```python
from build123d import *

# Parameters (mm, degrees)
F1_DEPTH = 12.7
F2_SIZE  = 2.54


with BuildPart() as f1:
    # F0 (on Top) → F1 (new body)
    with BuildSketch(Plane.XY):
        Polygon((0, 76.2), (0, 0), (50.8, 0), (50.8, 55.88), (25.4, 76.2), align=None)
        Polygon((-50.8, 0), (0, 0), (0, 76.2), (-25.4, 76.2), (-50.8, 55.88), align=None)
        Polygon((0, -76.2), (0, 0), (-50.8, 0), (-50.8, -55.88), (-25.4, -76.2), align=None)
        Polygon((50.8, 0), (0, 0), (0, -76.2), (25.4, -76.2), (50.8, -55.88), align=None)
    extrude(amount=F1_DEPTH)

    # F2
    f2_edges = [f1.edges().sort_by_distance(p)[0] for p in [
        (50.8, 0, 0),
        (38.1, 66.04, 0),
        (0, 76.2, 0),
        (-38.1, 66.04, 0),
        (-50.8, 0, 0),
        (-38.1, -66.04, 0),
        (0, -76.2, 0),
        (38.1, -66.04, 0),
    ]]
    chamfer(f2_edges, length=F2_SIZE)


solid = f1.part
```
Input: part model. Units: mm. Frame: model coordinates. Coordinates: 2 decimals unless noted, no trailing zeros. Write each loop counter-clockwise with the first axis right and the second up, starting at its lowest first coordinate (ties: lowest second). Pieces come first, ordered by that corner, then holes. Notation, with made-up numbers: (80, -0.5) - (108, -0.5) arc R16 ccw to (108, 13.5) - close; hole circle Ø5 at (41, 37.25). An arc over 180 degrees is marked (long way). Put each result on its own line as item: value. Start each with the question number.
1) Cut plane A-A (z = 8). Return the cut outline in (x, y).
2) Cut plane C-C (y = -63.5). Return the cut outline in (x, z) (3 decimals), plus the area to 3 significant figures.
3) Cut plane B-B (x = 42). Return the cut outline in (y, z), plus the area to 3 significant figures.
4) Ray query, L1, parallel to X at y = -29, z = 0.5; L2, parallel to X at y = 69, z = 1.5; L3, parallel to Y at x = -25.5, z = 9.5. Return the intervals inside material, ascending.
5) Contact query for flat-ended pins moving along their axis: pin 1 (1 mm diameter, centred on x = 36.5, z = 7.5, fed in from -Y); pin 2 (5 mm diameter, centred on x = -40.5, z = 2.5, fed in from +Y). Output: stop coordinate, or through.
Resolved:
1. outline: (-50.8, -55.88) - (-25.4, -76.2) - (25.4, -76.2) - (50.8, -55.88) - (50.8, 55.88) - (25.4, 76.2) - (-25.4, 76.2) - (-50.8, 55.88) - close
2. outline: (-41.275, 2.54) - (-37.209, 0) - (37.209, 0) - (41.275, 2.54) - (41.275, 12.7) - (-41.275, 12.7) - close
2. area: 1,040 mm2
3. outline: (-62.92, 2.54) - (-59.67, 0) - (59.67, 0) - (62.92, 2.54) - (62.92, 12.7) - (-62.92, 12.7) - close
3. area: 1,590 mm2
4. L1: x = -48.76 to 48.76
4. L2: x = -32.74 to 32.74
4. L3: y = -76.12 to 76.12
5. pin 1: stops at y = -67.72
5. pin 2: stops at y = 66.12
